from build123d import *

# Parameters (mm, degrees)
SKETCH1_R           = 25
SKETCH1_R_2         = 12.5
SKETCH1_R_3         = 2
BOSS_EXTRUDE1_DEPTH = 14.5
CHAMFER1_SIZE       = 3


with BuildPart() as part:
    # Sketch1 → Boss-Extrude1 (new body)
    with BuildSketch(Plane.XY):
        Circle(SKETCH1_R)
        Circle(SKETCH1_R_2, mode=Mode.SUBTRACT)
        with Locations((0, 18)):
            Circle(SKETCH1_R_3, mode=Mode.SUBTRACT)
        with Locations((9, 15.588457268)):
            Circle(SKETCH1_R_3, mode=Mode.SUBTRACT)
        with Locations((18, 0)):
            Circle(SKETCH1_R_3, mode=Mode.SUBTRACT)
        with Locations((9, -15.588457268)):
            Circle(SKETCH1_R_3, mode=Mode.SUBTRACT)
        with Locations((0, -18)):
            Circle(SKETCH1_R_3, mode=Mode.SUBTRACT)
        with Locations((-9, -15.588457268)):
            Circle(SKETCH1_R_3, mode=Mode.SUBTRACT)
        with Locations((-18, 0)):
            Circle(SKETCH1_R_3, mode=Mode.SUBTRACT)
        with Locations((-9, 15.588457268)):
            Circle(SKETCH1_R_3, mode=Mode.SUBTRACT)
    extrude(amount=BOSS_EXTRUDE1_DEPTH)

    # Chamfer1
    chamfer1_edges = [part.edges().sort_by_distance(p)[0] for p in [
        (-25, 0, 14.5),
    ]]
    chamfer(chamfer1_edges, length=CHAMFER1_SIZE)


solid = part.part
For this review, take the finished solid that the model builds, in its own axes (mm). Coordinates: 2 decimals unless noted, no trailing zeros. Loops run counter-clockwise (first coordinate to the right, second up) from the corner with the lowest first, then second, coordinate; pieces in that order, holes last. Notation, with made-up numbers: (43.5, 45) -> (61.5, 45) arc R10 ccw to (61.5, 58) -> close; hole circle Ø6 at (27, 35.25). An arc over 180 degrees is marked (long way). Write each question's results on one line, items separated by ' | '.
Q1. To check wall thickness, follow line 1 along Y through (x, z) = (0, 3.5); line 2 along Y through (x, z) = (-9, 4.5); line 3 along Y through (x, z) = (-2.5, 11.25). State the ranges of each line that lie inside material, in increasing order. Write a range as [from, to].
Taken from the geometry:
line 1: [-25, -20], [-16, -12.5], [12.5, 16], [20, 25] | line 2: [-23.32, -17.59], [-13.59, -8.67], [8.67, 13.59], [17.59, 23.32] | line 3: [-24.87, -12.25], [12.25, 24.87]
Q2. Mouldability with a two-part tool opening along Y and no side actions: class faces 1 (the flat face through (-5.9, 11.5, 0)), 2 (the cylindrical face through (11.923, 3.755, 7.148)), 3 (the conical face through (-4.801, -21.619, 14.354)) as +Y half, -Y half, draft (parallel to the pull), parting line (faces both ways), or undercut.
Taken from the geometry:
face 1: draft | face 2: undercut | face 3: parting line
Q3. Add section C-C, the plane z = 5.25. Count the separate pieces of the cut face and the enclosed holes in it, then the cut area to 3 significant figures.
Taken from the geometry:
separate pieces: 1 | enclosed holes: 9 | area: 1,370 mm²
Q4. Add section A-A, the plane y = 0. State the section outline as (x, z) points, then the cut area to 4 significant figures.
Taken from the geometry:
outline: (-25, 0) -> (-20, 0) -> (-20, 14.5) -> (-22, 14.5) -> (-25, 11.5) -> close; (-16, 0) -> (-12.5, 0) -> (-12.5, 14.5) -> (-16, 14.5) -> close; (12.5, 0) -> (16, 0) -> (16, 14.5) -> (12.5, 14.5) -> close; (20, 0) -> (25, 0) -> (25, 11.5) -> (22, 14.5) -> (20, 14.5) -> close | area: 237.5 mm²
Q5. For pin 1 Ø6 at (x, z) = (-19, 4.5) entering from +Y; pin 2 Ø3 at (x, y) = (9, 15.59) entering from +Z; pin 3 Ø3 at (y, z) = (-7.5, 3.5) entering from +X; pin 4 Ø1.5 at (x, z) = (-1, 12.5) entering from +Y, all flat-tipped, find the tip position at first contact; note any pin that passes through.
Taken from the geometry:
pin 1: y = 19.21 | pin 2: through | pin 3: x = 24.27 | pin 4: y = 24.73
